The figure shows three views and two pictorial views of one solid part (mm, origin at its lowest corner). Answer the questions. A direction names the side the tool comes from. Give positions to 0.01 mm unless a question says otherwise; leave off trailing zeros. Loops run counter-clockwise (first coordinate to the right, second up) from the corner with the lowest first, then second, coordinate; pieces in that order, holes last. Notation, with made-up numbers: (13.25, 35.5) - (54.25, 35.5) arc R17 cw to (54.25, 49.5) - close; hole circle Ø8 at (46.5, -39). An arc over 180 degrees is marked (long way). Write item = value, one per line.
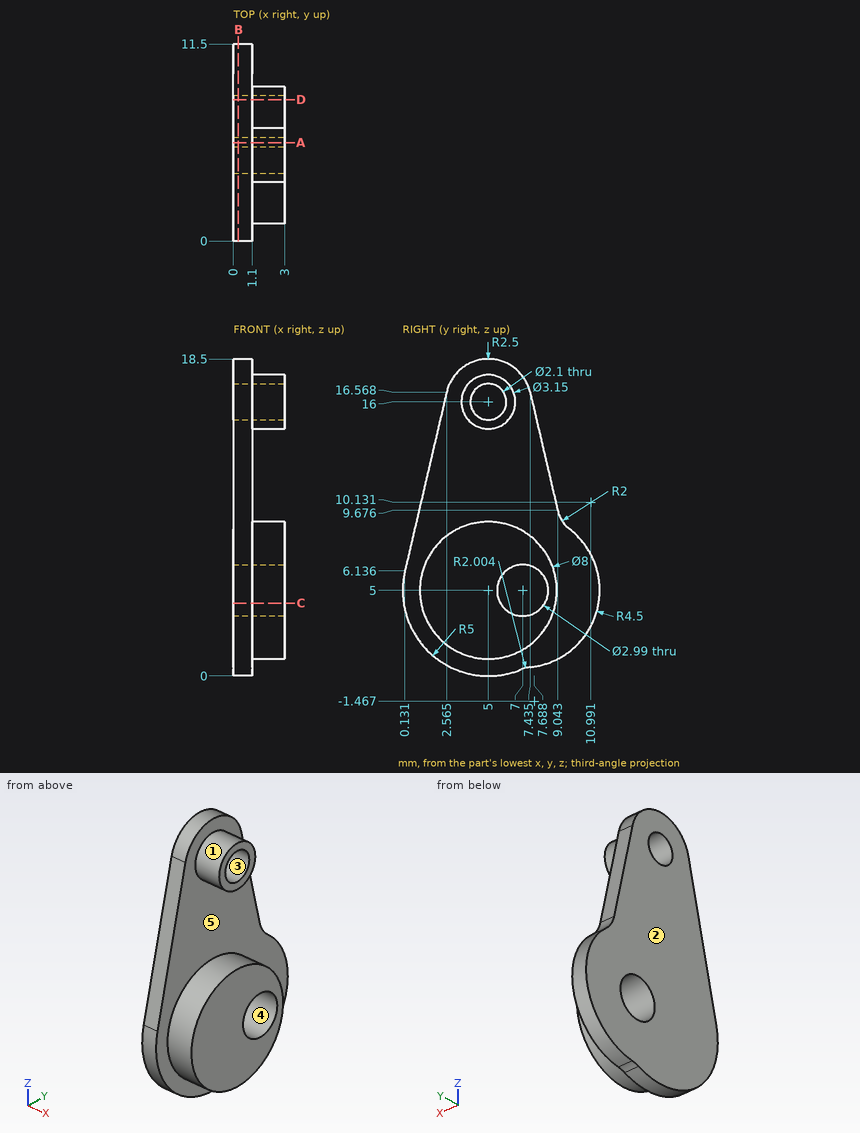
1) A cutting plane is placed at D-D on y = 8.25. Determine the outline of the cut face in (x, z) (1 decimal).
Output:
outline = (0, 0.7) - (1.1, 0.7) - (1.1, 2.7) - (3, 2.7) - (3, 4.2) - (0, 4.2) - close; (0, 5.8) - (3, 5.8) - (3, 7.3) - (1.1, 7.3) - (1.1, 13.1) - (0, 13.1) - close
2) Find the intervals of material crossed by probe 1 along X at (y, z) = (4.5, 12.75); probe 2 along Z at (x, y) = (0.4, 5.75) (1 decimal); probe 3 along Y at (x, z) = (0.35, 16), in increasing order.
Output:
probe_1 = 0 to 1.1
probe_2 = 0.1 to 4.2, 5.8 to 15.3, 16.7 to 18.4
probe_3 = 2.43 to 3.95, 6.05 to 7.57
3) A tool of negligible diameter and unlimited length cuts with its end or side. For the marked faces 4 and 5, from which of +Z, -Z, +X, -X, +Y, -Y can it reach the whole face along a straight path? Write none if from no direction.
Output:
face_4 = +X, -X
face_5 = +X
4) A cutting plane is placed at C-C on z = 4.25. Determine the outline of the cut face in (x, y).
Output:
outline = (0, 0.06) - (1.1, 0.06) - (1.1, 1.07) - (3, 1.07) - (3, 5.71) - (0, 5.71) - close; (0, 8.29) - (3, 8.29) - (3, 8.93) - (1.1, 8.93) - (1.1, 11.44) - (0, 11.44) - close
5) The mould has two halves that part along Y. Classify the marked faces 1, 2 and 3: pulls with the +Y half, pulls with the -Y half, needs draft (parallel to the pull), parting line crosses it, or undercut.
Output:
face_1 = parting line crosses it
face_2 = needs draft
face_3 = undercut
6) A cutting plane is placed at B-B on x = 0.3. Give the number of separate pieces and of enclosed holes in the cut face, then the cut area to 3 significant figures.
Output:
separate_pieces = 1
enclosed_holes = 2
area = 134 mm²
7) A cutting plane is placed at A-A on y = 5.75. Determine the outline of the cut face in (x, z) (1 decimal).
Output:
outline = (0, 0.1) - (1.1, 0.1) - (1.1, 1.1) - (3, 1.1) - (3, 4.2) - (0, 4.2) - close; (0, 5.8) - (3, 5.8) - (3, 8.9) - (1.1, 8.9) - (1.1, 14.6) - (3, 14.6) - (3, 15.3) - (0, 15.3) - close; (0, 16.7) - (3, 16.7) - (3, 17.4) - (1.1, 17.4) - (1.1, 18.4) - (0, 18.4) - close
